Could you check a few things on this model? Use its own coordinates, in mm. Face numbers are marked on the shaded views. A direction names the side the tool comes from. Give positions to 0.01 mm unless a question says otherwise; leave off trailing zeros. Order: outer loops, then holes, each group sorted by start corner. A loop starts at its lowest first (then second) coordinate and runs counter-clockwise, first axis right, second up. Notation, with made-up numbers: (17, 68) -> (41, 68) arc R27 cw to (41, 87) -> close; hole circle Ø1 at (74.25, -2). An arc over 180 degrees is marked (long way). Answer as CSV lines item,"result". Start each with the question number.
(1) We'd pull the mould along Z, two halves only. Please class the marked faces 3, 4 and 5: released by +Z, released by -Z, zero draft, split by the parting line, or undercut.
(2) I want a section at A-A (z = 0). Please give me the cut outline in (x, y), plus the area to 3 significant figures.
(3) On a 3-axis mill with a long thin cutter (end or side, diameter ignored), from which of +Z, -Z, +X, -X, +Y, -Y can I reach the whole of each face in a straight line? I mean the marked faces 1 and 2. Say none if no direction works.
(4) Will these pins go through, and if not, where does the flat tip stop? pin 1 Ø8 at (x, z) = (-5.5, -10.5) entering from -Y; pin 2 Ø1.5 at (x, y) = (-0.5, 25) entering from -Z; pin 3 Ø2 at (y, z) = (15, 1.5) entering from -X.
(5) I need wall thicknesses on L1, parallel to X at y = 3.25, z = 0; L2, parallel to Y at x = -12, z = -8.5; L3, parallel to Z at x = -2, y = 13.75. Which ranges of each line are inside material? Lowest first, please.
(6) I want a section at B-B (y = 5.5). Please give me the cut outline in (x, z).
(7) I want a section at C-C (y = 13.75). Please give me the cut outline in (x, z), plus the area to 3 significant figures.
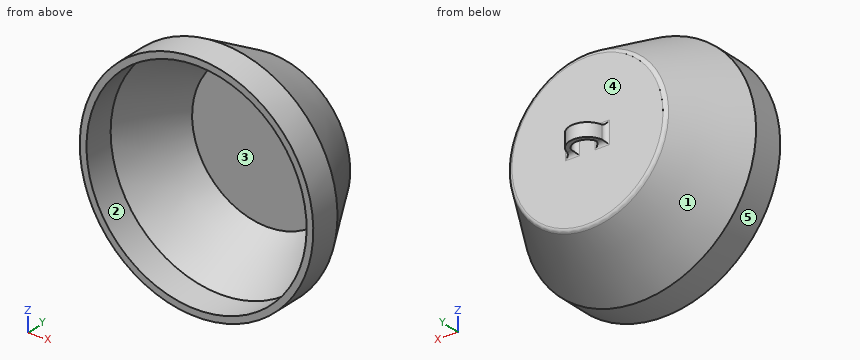
```python
from build123d import *

# Parameters (mm, degrees)
SKETCH1_R           = 26.15
SKETCH1_R_2         = 24.65
BOSS_EXTRUDE1_DEPTH = 7
SKETCH3_R           = 26.15
BOSS_EXTRUDE2_DEPTH = 15
BOSS_EXTRUDE2_TAPER = 30
SKETCH4_R           = 24.65
CUT_EXTRUDE1_DEPTH  = 13.5
CUT_EXTRUDE1_DRAFT  = -30
BOSS_EXTRUDE4_DEPTH = 1.5
FILLET2_R           = 1


with BuildPart() as part:
    # Sketch1 → Boss-Extrude1 (new body)
    with BuildSketch(Plane(origin=(0, 0, 0), x_dir=(1, 0, 0), z_dir=(0, 1, 0))):
        with Locations(Location((0, 0, 0), (0, 0, 270))):
            Circle(SKETCH1_R)
        with Locations(Location((0, 0, 0), (0, 0, 270))):
            Circle(SKETCH1_R_2, mode=Mode.SUBTRACT)
    extrude(amount=BOSS_EXTRUDE1_DEPTH)

    # Sketch3 → Boss-Extrude2 (add)
    with BuildSketch(Plane(origin=(0, 7, 0), x_dir=(1, 0, 0), z_dir=(0, 1, 0))):
        with Locations(Location((0, 0, 0), (0, 0, 270))):
            Circle(SKETCH3_R)
    extrude(amount=BOSS_EXTRUDE2_DEPTH, taper=BOSS_EXTRUDE2_TAPER)


with BuildPart() as cut_extrude1_tool:
    # Sketch4 → Cut-Extrude1 (with draft: the straight prism first)
    with BuildSketch(Plane.XZ.offset(-7)):
        with Locations(Location((0, 0, 0), (0, 0, 270))):
            Circle(SKETCH4_R)
    extrude(amount=-CUT_EXTRUDE1_DEPTH)
    # Cut-Extrude1: the draft: its side faces are tilted about the plane it starts from
    cut_extrude1_sides = [cut_extrude1_tool.faces().sort_by_distance(p)[0] for p in [
        (0, 13.75, 24.65),
    ]]
    draft(cut_extrude1_sides, Plane.XZ.offset(-7), CUT_EXTRUDE1_DRAFT)


with BuildPart() as part_1:
    add(part.part)

    # Cut-Extrude1: cut by cut_extrude1_tool
    add(cut_extrude1_tool.part, mode=Mode.SUBTRACT)

    # Sketch5 → Boss-Extrude4 (add, symmetric)
    with BuildSketch(Plane.XY):
        with BuildLine():
            Line((-4, 22), (-3, 22))
            ThreePointArc((-3, 22), (0, 25), (3, 22))
            Line((3, 22), (4, 22))
            ThreePointArc((4, 22), (0, 26), (-4, 22))
        make_face()
    extrude(amount=BOSS_EXTRUDE4_DEPTH, both=True)

    # Fillet2
    fillet2_edges = [part_1.edges().sort_by_distance(p)[0] for p in [
        (0, 22, -17.489745962),
        (4, 22, 0),
        (-3.5, 22, -1.5),
        (-4, 22, 0),
        (-3, 22, 0),
        (3.5, 22, -1.5),
        (3, 22, 0),
        (-3.5, 22, 1.5),
        (3.5, 22, 1.5),
    ]]
    fillet(fillet2_edges, radius=FILLET2_R)


solid = part_1.part
```
Final values:
1,face 3,"undercut"
1,face 4,"zero draft"
1,face 5,"split by the parting line"
2,outline,"(-26.15, 0) -> (-24.65, 0) -> (-24.65, 7) -> (-16.86, 20.5) -> (16.86, 20.5) -> (24.65, 7) -> (24.65, 0) -> (26.15, 0) -> (26.15, 7) -> (17.78, 21.5) arc R1 ccw to (16.91, 22) -> (4.9, 22) arc R1 cw to (3.92, 22.8) arc R4 ccw to (-3.92, 22.8) arc R1 cw to (-4.9, 22) -> (-16.91, 22) arc R1 ccw to (-17.78, 21.5) -> (-26.15, 7) -> close; hole (-2.6, 23.5) arc R1 ccw to (-1.73, 22) -> (1.73, 22) arc R1 ccw to (2.6, 23.5) arc R3 ccw to start"
2,area,"127 mm²"
3,face 1,"+Y"
3,face 2,"-Y"
4,pin 1,"y = 20.5"
4,pin 2,"z = -1.5"
4,pin 3,"x = -22.06"
5,L1,"-26.15 to -24.65, 24.65 to 26.15"
5,L2,"20.5 to 22"
5,L3,"-22.16 to -20.66, 20.66 to 22.16"
6,outline,"circle Ø52.3 at (0, 0); hole circle Ø49.3 at (0, 0)"
7,outline,"circle Ø44.51 at (0, 0); hole circle Ø41.51 at (0, 0)"
7,area,"203 mm²"
